Input: part model. Units: mm. Frame: model coordinates. Face numbers are marked on the shaded views. A direction names the side the tool comes from. Coordinates: 2 decimals unless noted, no trailing zeros. Loops run counter-clockwise (first coordinate to the right, second up) from the corner with the lowest first, then second, coordinate; pieces in that order, holes last.
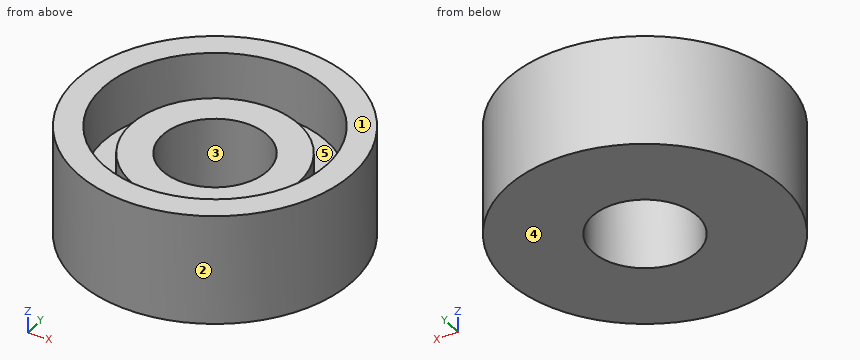
```python
from build123d import *

# Parameters (mm, degrees)
F0_R      = 5
F1_DEPTH  = 4
F2_R      = 4.064
F2_R_2    = 3.048
F3_DEPTH  = 2
F3_FACE_R = 3.048
F4_DEPTH  = 1
F5_R      = 1.905
F6_DEPTH  = 25.4


with BuildPart() as f1:
    # F0 (on Top) → F1 (new body)
    with BuildSketch(Plane.XY):
        Circle(F0_R)
    extrude(amount=F1_DEPTH)

    # F2 (on face) → F3 (cut)
    with BuildSketch(Plane.XY.offset(4)):
        Circle(F2_R)
        Circle(F2_R_2, mode=Mode.SUBTRACT)
    extrude(amount=-F3_DEPTH, mode=Mode.SUBTRACT)

    # F3_face (on face) → F4 (cut)
    with BuildSketch(Plane.XY.offset(4)):
        Circle(F3_FACE_R)
    extrude(amount=-F4_DEPTH, mode=Mode.SUBTRACT)

    # F5 (on face) → F6 (cut)
    with BuildSketch(Plane.XY.offset(3)):
        Circle(F5_R)
    extrude(amount=-F6_DEPTH, mode=Mode.SUBTRACT)


solid = f1.part
```
Item 1: Line query: L1, parallel to Y at x = 0, z = 0.95 (3 decimals); L2, parallel to X at y = 0.5, z = 2.75; L3, parallel to Z at x = -1.75, y = -3.25. Output: solid intervals per line, ascending.
Result:
L1: y = -5 to -1.905, 1.905 to 5
L2: x = -4.97 to -4.03, -3.01 to -1.84, 1.84 to 3.01, 4.03 to 4.97
L3: z = 0 to 2
Item 2: Reachability of the marked faces 4 and 5 from +Z, -Z, +X, -X, +Y, -Y: full face, straight path, thin tool, end or side. Return the list, or none.
Result:
face 4: -Z, +X, -X, +Y, -Y
face 5: +Z
Item 3: Section query D-D (z = 0.95). Output: boundary loops of the cut face in (x, y) (3 decimals).
Result:
outline: circle Ø10 at (0, 0); hole circle Ø3.81 at (0, 0)
Item 4: Section query C-C (z = 2.15). Output: boundary loops of the cut face in (x, y) (3 decimals), then the cut area to 3 significant figures.
Result:
outline: circle Ø10 at (0, 0); circle Ø6.096 at (0, 0); hole circle Ø8.128 at (0, 0); hole circle Ø3.81 at (0, 0)
area: 44.4 mm2
Item 5: Contact query for a flat-ended pin moving along its axis: P1, Ø1, axis at x = 3.5, z = 3, coming from the +Y side. Output: stop coordinate, or through.
Result:
P1: stops at y = 4
Item 6: Section query A-A (x = 0). Output: boundary loops of the cut face in (y, z) (3 decimals).
Result:
outline: (-5, 0) - (-1.905, 0) - (-1.905, 3) - (-3.048, 3) - (-3.048, 2) - (-4.064, 2) - (-4.064, 4) - (-5, 4) - close; (1.905, 0) - (5, 0) - (5, 4) - (4.064, 4) - (4.064, 2) - (3.048, 2) - (3.048, 3) - (1.905, 3) - close
Item 7: Mould query, pull axis X, two halves, no side actions, for the marked faces 1, 2 and 3. Classes: +X half, -X half, draft (parallel to the pull), parting line (faces both ways), or undercut.
Result:
face 1: draft
face 2: parting line
face 3: undercut
